Source: CAD feature listing. Evaluate the final solid. Frame: model axes, mm. A direction names the side the tool comes from. Round coordinates to 2 decimals unless told otherwise and drop trailing zeros. Loops run counter-clockwise (first coordinate to the right, second up) from the corner with the lowest first, then second, coordinate; pieces in that order, holes last.
(1) Section A-A, the plane z = 5. Return the cut outline in (x, y).
(2) Section C-C, the plane y = 28. Return the cut outline in (x, z), plus the area to 3 significant figures.
(3) Section D-D, the plane x = 51.5. Return the cut outline in (y, z), plus the area to 3 significant figures.
(4) Section B-B, the plane z = 35.5. Return the cut outline in (x, y), plus the area to 3 significant figures.
(5) Mould query, pull axis Z, two halves, no side actions, for faces 4 (the flat face through (-9, 14, 0)), 5 (the flat face through (-47.5, 45.5, 25)), 6 (the flat face through (24.1, 0, 55.4)). Classes: pulls with the +Z half, pulls with the -Z half, needs draft (parallel to the pull), parting line crosses it, or undercut.
(6) First-contact query: pin 1 Ø2 at (y, z) = (50, 22.5) entering from -X; pin 2 Ø22.5 at (x, y) = (-41.56, 34) entering from -Z; pin 3 Ø4 at (y, z) = (2.5, 55) entering from -X; pin 4 Ø17 at (x, y) = (-2, 21.5) entering from +Z. Flat tips, straight axial feed; report the tip coordinate or a pass-through.
(7) Material intervals for probe 1 along Z at (x, y) = (46, -1.5); probe 2 along Z at (x, y) = (8.5, 2.5); probe 3 along Y at (x, z) = (74, 27), sorted ascending.
(8) Set-up query: faces 1 (the flat face through (31, 1, 23.242)), 2 (the cylindrical face through (55.72, -6.63, 39.07)), 3 (the flat face through (32, 1, 55.242)). Return all of +Z, -Z, +X, -X, +Y, -Y with unobstructed straight access to the full face (end or side cutting, diameter ignored); none if empty.
```python
from build123d import *

# Parameters (mm, degrees)
SKETCH1_R           = 12.5
SKETCH1_W           = 150
SKETCH1_H           = 16
BOSS_EXTRUDE4_DEPTH = 16
SKETCH6_R           = 25
SKETCH6_R_2         = 12.5
BOSS_EXTRUDE5_DEPTH = 9
BOSS_EXTRUDE6_DEPTH = 16
CUT_EXTRUDE2_DEPTH  = 17
BOSS_EXTRUDE7_DEPTH = 3
CUT_EXTRUDE6_DEPTH  = 60


with BuildPart() as part:
    # Sketch1 → Boss-Extrude4 (new body)
    with BuildSketch(Plane.XY):
        with BuildLine():
            ThreePointArc((-31.360767673, 56.826225363), (-55.160209154, 54.975058449), (-66.55701383, 34))
            ThreePointArc((-66.55701383, 34), (-41.55701383, 9), (-16.55701383, 34))
            ThreePointArc((-16.55701383, 34), (-20.060743341, 46.763634086), (-29.589842236, 55.949642459))
            Line((-29.589842236, 55.949642459), (-31.360767673, 56.826225363))
        make_face()
        with Locations((-41.55701383, 34)):
            Circle(SKETCH1_R, mode=Mode.SUBTRACT)
        with BuildLine():
            Line((-66.55701383, 34), (-66.55701383, 0))
            Line((-66.55701383, 0), (83.44298617, 0))
            Line((83.44298617, 0), (-29.589842236, 55.949642459))
            ThreePointArc((-29.589842236, 55.949642459), (-20.060743341, 46.763634086), (-16.55701383, 34))
            ThreePointArc((-16.55701383, 34), (-41.55701383, 9), (-66.55701383, 34))
        make_face()
        with Locations((8.44298617, -8)):
            Rectangle(SKETCH1_W, SKETCH1_H)
    extrude(amount=BOSS_EXTRUDE4_DEPTH)

    # Sketch6 → Boss-Extrude5 (add)
    with BuildSketch(Plane.XY.offset(16)):
        with Locations((-41.55701383, 34)):
            Circle(SKETCH6_R)
        with Locations((-41.55701383, 34)):
            Circle(SKETCH6_R_2, mode=Mode.SUBTRACT)
    extrude(amount=BOSS_EXTRUDE5_DEPTH)

    # Sketch7 → Boss-Extrude6 (add)
    with BuildSketch(Plane.XZ.offset(16)):
        Polygon((83.44298617, 16), (83.44298617, 70), (8.44298617, 70), (-66.55701383, 16), align=None)
    extrude(amount=-BOSS_EXTRUDE6_DEPTH)

    # Sketch8 → Cut-Extrude2 (cut, through all)
    with BuildSketch(Plane(origin=(0, 0, 0), x_dir=(1, 0, 0), z_dir=(0, 1, 0))):
        with BuildLine():
            Line((47.721749713, -47.241556866), (15.721749713, -47.241556866))
            ThreePointArc((15.721749713, -47.241556866), (7.721749713, -39.241556866), (15.721749713, -31.241556866))
            Line((15.721749713, -31.241556866), (47.721749713, -31.241556866))
            ThreePointArc((47.721749713, -31.241556866), (55.721749713, -39.241556866), (47.721749713, -47.241556866))
        make_face()
    extrude(amount=-CUT_EXTRUDE2_DEPTH, mode=Mode.SUBTRACT)

    # Sketch9 → Boss-Extrude7 (add)
    with BuildSketch(Plane(origin=(0, 0, 0), x_dir=(1, 0, 0), z_dir=(0, 1, 0))):
        with BuildLine():
            Line((47.721749713, -55.241556866), (15.721749713, -55.241556866))
            ThreePointArc((15.721749713, -55.241556866), (-0.278250287, -39.241556866), (15.721749713, -23.241556866))
            Line((15.721749713, -23.241556866), (47.721749713, -23.241556866))
            ThreePointArc((47.721749713, -23.241556866), (63.721749713, -39.241556866), (47.721749713, -55.241556866))
        make_face()
    extrude(amount=BOSS_EXTRUDE7_DEPTH)

    # Sketch10 → Cut-Extrude6 (cut, through all)
    with BuildSketch(Plane(origin=(0, 0, 0), x_dir=(1, 0, 0), z_dir=(0, 1, 0))):
        with BuildLine():
            Line((47.721749713, -47.241556866), (15.721749713, -47.241556866))
            ThreePointArc((15.721749713, -47.241556866), (7.721749713, -39.241556866), (15.721749713, -31.241556866))
            Line((15.721749713, -31.241556866), (47.721749713, -31.241556866))
            ThreePointArc((47.721749713, -31.241556866), (55.721749713, -39.241556866), (47.721749713, -47.241556866))
        make_face()
    extrude(amount=CUT_EXTRUDE6_DEPTH, mode=Mode.SUBTRACT)


solid = part.part
```
Output values:
1. outline: (-66.56, -16) - (83.44, -16) - (83.44, 0) - (-31.36, 56.83) arc R25 ccw to (-66.56, 34) - close; hole circle Ø25 at (-41.56, 34)
2. outline: (-66.56, 0) - (-52.52, 0) - (-52.52, 25) - (-65.83, 25) - (-65.83, 16) - (-66.56, 16) - close; (-30.59, 0) - (26.88, 0) - (26.88, 16) - (-17.29, 16) - (-17.29, 25) - (-30.59, 25) - close
2. area: 1,380 mm2
3. outline: (-16, 0) - (15.81, 0) - (15.81, 16) - (0, 16) - (0, 23.69) - (3, 23.69) - (3, 32.19) - (-16, 32.19) - close; (-16, 46.29) - (3, 46.29) - (3, 54.79) - (0, 54.79) - (0, 70) - (-16, 70) - close
3. area: 1,200 mm2
4. outline: (-39.47, -16) - (8.65, -16) - (8.65, 3) - (0.17, 3) - (0.17, 0) - (-39.47, 0) - close; (54.79, -16) - (83.44, -16) - (83.44, 0) - (63.28, 0) - (63.28, 3) - (54.79, 3) - close
4. area: 1,280 mm2
5. face 4: pulls with the -Z half
5. face 5: pulls with the +Z half
5. face 6: undercut
6. pin 1: stops at x = -61.56
6. pin 2: passes through
6. pin 3: stops at x = 7.55
6. pin 4: stops at z = 16
7. probe 1: z = 0 to 31.24, 47.24 to 70
7. probe 2: z = 0 to 16, 24.96 to 35.8, 42.68 to 53.52
7. probe 3: y = -16 to 0
8. face 1: +X, -X, +Y
8. face 2: +Y, -Y
8. face 3: +Z, +X, -X, +Y
